```python
from build123d import *

# Parameters (mm, degrees)
F0_W     = 100
F0_H     = 54
F0_R     = 2.25
F1_DEPTH = 2
F2_W     = 2
F2_H     = 2
F2_R     = 1.75
F3_DEPTH = 2
F4_R     = 3
F5_R     = 1.5


# Not quite as in the source:
# - a feature names something its author has since deleted; it is built from what else it names


with BuildPart() as f1:
    # F0 (on Front) → F1 (new body)
    with BuildSketch(Plane.XZ):
        with Locations((50, 27)):
            Rectangle(F0_W, F0_H)
        with Locations((5, 5)):
            Circle(F0_R, mode=Mode.SUBTRACT)
        with Locations((39, 5)):
            Circle(F0_R, mode=Mode.SUBTRACT)
        with Locations((61, 5)):
            Circle(F0_R, mode=Mode.SUBTRACT)
        with Locations((95, 5)):
            Circle(F0_R, mode=Mode.SUBTRACT)
        with Locations((5, 49)):
            Circle(F0_R, mode=Mode.SUBTRACT)
        with Locations((39, 49)):
            Circle(F0_R, mode=Mode.SUBTRACT)
        with Locations((61, 49)):
            Circle(F0_R, mode=Mode.SUBTRACT)
        with Locations((95, 49)):
            Circle(F0_R, mode=Mode.SUBTRACT)
    extrude(amount=F1_DEPTH)

    # F2 (on face) → F3 (cut)
    with BuildSketch(Plane.XZ.offset(2)):
        with Locations((24, 28)):
            Rectangle(F2_W, F2_H)
        with BuildLine():
            Line((23, 25), (23, 27))
            Line((23, 27), (23, 29))
            Line((23, 29), (17.5, 29))
            ThreePointArc((17.5, 29), (15.5, 27), (17.5, 25))
            Line((17.5, 25), (23, 25))
        make_face()
        with Locations((24, 26)):
            Rectangle(F2_W, F2_H)
        with Locations((26, 28)):
            Rectangle(F2_W, F2_H)
        with Locations((26, 26)):
            Rectangle(F2_W, F2_H)
        with BuildLine():
            Line((23, 34.5), (23, 29))
            Line((23, 29), (25, 29))
            Line((25, 29), (27, 29))
            Line((27, 29), (27, 34.5))
            ThreePointArc((27, 34.5), (25, 36.5), (23, 34.5))
        make_face()
        with BuildLine():
            Line((25, 25), (23, 25))
            Line((23, 25), (23, 19.5))
            ThreePointArc((23, 19.5), (25, 17.5), (27, 19.5))
            Line((27, 19.5), (27, 25))
            Line((27, 25), (25, 25))
        make_face()
        with BuildLine():
            Line((27, 29), (27, 27))
            Line((27, 27), (27, 25))
            Line((27, 25), (32.5, 25))
            ThreePointArc((32.5, 25), (34.5, 27), (32.5, 29))
            Line((32.5, 29), (27, 29))
        make_face()
        with Locations((50, 27)):
            Circle(F2_R)
        with Locations((74, 28)):
            Rectangle(F2_W, F2_H)
        with BuildLine():
            Line((73, 25), (73, 27))
            Line((73, 27), (73, 29))
            Line((73, 29), (67.5, 29))
            ThreePointArc((67.5, 29), (65.5, 27), (67.5, 25))
            Line((67.5, 25), (73, 25))
        make_face()
        with Locations((74, 26)):
            Rectangle(F2_W, F2_H)
        with Locations((76, 28)):
            Rectangle(F2_W, F2_H)
        with Locations((76, 26)):
            Rectangle(F2_W, F2_H)
        with BuildLine():
            Line((73, 34.5), (73, 29))
            Line((73, 29), (75, 29))
            Line((75, 29), (77, 29))
            Line((77, 29), (77, 34.5))
            ThreePointArc((77, 34.5), (75, 36.5), (73, 34.5))
        make_face()
        with BuildLine():
            Line((75, 25), (73, 25))
            Line((73, 25), (73, 19.5))
            ThreePointArc((73, 19.5), (75, 17.5), (77, 19.5))
            Line((77, 19.5), (77, 25))
            Line((77, 25), (75, 25))
        make_face()
        with BuildLine():
            Line((77, 29), (77, 27))
            Line((77, 27), (77, 25))
            Line((77, 25), (82.5, 25))
            ThreePointArc((82.5, 25), (84.5, 27), (82.5, 29))
            Line((82.5, 29), (77, 29))
        make_face()
    extrude(amount=-F3_DEPTH, mode=Mode.SUBTRACT)

    # F4
    f4_edges = [f1.edges().sort_by_distance(p)[0] for p in [
        (23, -1, 29),
        (23, -1, 25),
        (27, -1, 25),
        (27, -1, 29),
        (73, -1, 29),
        (77, -1, 29),
        (77, -1, 25),
        (73, -1, 25),
    ]]
    fillet(f4_edges, radius=F4_R)

    # F5
    f5_edges = [f1.edges().sort_by_distance(p)[0] for p in [
        (0, -1, 54),
        (0, -1, 0),
        (100, -1, 54),
        (100, -1, 0),
    ]]
    fillet(f5_edges, radius=F5_R)


solid = f1.part
```
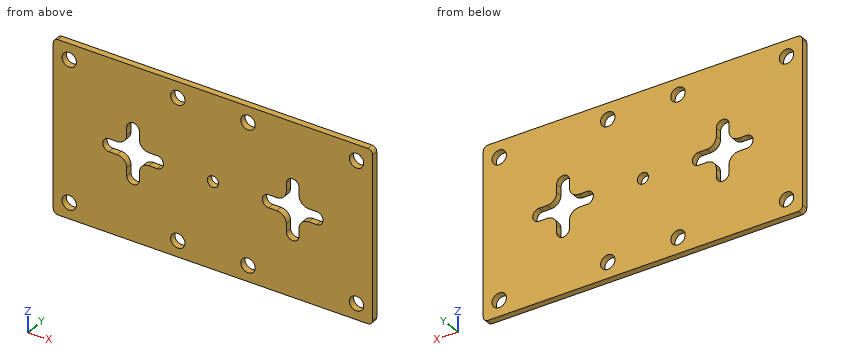
Part model, mm, in its own coordinate system. Round coordinates to 2 decimals unless told otherwise and drop trailing zeros. Order: outer loops, then holes, each group sorted by start corner. A loop starts at its lowest first (then second) coordinate and runs counter-clockwise, first axis right, second up. Notation, with made-up numbers: M 58.25,-17.75 L 87.25,-17.75 A21 cw 87.25,-5.75 Z; hole C 34,25.25 d6. An arc over 180 degrees is marked long. Put each result on its own line as item: value. Start each with the question number.
1. Drop a flat-ended pin along its axis: pin 1 (2.5 mm diameter, centred on x = 39, z = 49, fed in from -Y). Give the stop position or say it passes through.
2. Slice it at B-B on x = 61. List the corners of the cut face in (y, z).
3. Slice it at C-C on x = 25. List the corners of the cut face in (y, z).
4. Slice it at D-D on y = -1.2. State how many separate pieces and enclosed holes the cut face has, then the cut area to 3 significant figures.
5. Drill centre lines: probe 1 along Z at (x, y) = (19, -1.8); probe 2 along Z at (x, y) = (94, -1.8); probe 3 along X at (y, z) = (-0.7, 30.5). Where is each one in solid material? Low to high. Write a range as [from, to].
6. Slice it at A-A on z = 5. List the corners of the cut face in (x, y).
Findings:
1. pin 1: through
2. outline: M -2,0 L 0,0 L 0,2.75 L -2,2.75 Z; M -2,7.25 L 0,7.25 L 0,46.75 L -2,46.75 Z; M -2,51.25 L 0,51.25 L 0,54 L -2,54 Z
3. outline: M -2,0 L 0,0 L 0,17.5 L -2,17.5 Z; M -2,36.5 L 0,36.5 L 0,54 L -2,54 Z
4. separate pieces: 1
4. enclosed holes: 11
4. area: 4,990 mm2
5. probe 1: [0, 25], [29, 54]
5. probe 2: [0, 2.98], [7.02, 46.98], [51.02, 54]
5. probe 3: [0, 22.6], [27.4, 72.6], [77.4, 100]
6. outline: M 0,-2 L 2.75,-2 L 2.75,0 L 0,0 Z; M 7.25,-2 L 36.75,-2 L 36.75,0 L 7.25,0 Z; M 41.25,-2 L 58.75,-2 L 58.75,0 L 41.25,0 Z; M 63.25,-2 L 92.75,-2 L 92.75,0 L 63.25,0 Z; M 97.25,-2 L 100,-2 L 100,0 L 97.25,0 Z
